Autodesk Inventor part; units mm, degrees
ref_plane "YZ Plane" through (0, 0, 0) normal (1, 0, 0) x (0, 1, 0)
ref_plane "XZ Plane" through (0, 0, 0) normal (0, 1, 0) x (-1, 0, 0)
ref_plane "XY Plane" through (0, 0, 0) normal (0, 0, 1) x (1, 0, 0)
sketch "Sketch1" plane through (0, 0, 0) normal (0, 1, 0) x (-1, 0, 0)
  line L0 (69.85, 63.5) -> (-82.55, 63.5)
  line L1 (-82.55, 63.5) -> (-82.55, -38.1)
  line L2 (-82.55, -38.1) -> (69.85, -38.1)
  line L3 (69.85, -38.1) -> (69.85, 63.5)
  circle A0 centre (25.4, -25.4) radius 3.9751
  circle A1 centre (63.5, 38.1) radius 3.175
  circle A2 centre (-76.2, 38.1) radius 3.175
  point P0 (0, 0)
  dimension "d0" = 101.6
  dimension "d1" = 152.4
  dimension "d3" = 38.1
  dimension "d4" = 7.9502
  dimension "d16" = 6.35
  dimension "d17" = 6.35
  dimension "d18" = 25.4
  dimension "d20" = 6.35
  dimension "d21" = 6.35
  dimension "d22" = 44.45
  dimension "d24" = 25.4
  dimension "d26" = 25.4
extrude "Extrusion1" add sketch "Sketch1" along normal blind 25.4
sketch "Sketch2" plane through (0, 25.4, 0) normal (0, 1, 0) x (1, 0, 0)
  circle A0 centre (6.35, -38.1) radius 16.51
  circle A1 centre (76.2, -38.1) radius 3.175
  line L0 (82.55, -63.5) -> (82.55, 38.1)
  point P0 (0, 0)
  dimension "d7" = 33.02
  dimension "d25" = 76.2
extrude "Extrusion2" add sketch "Sketch2" along normal blind 101.6 contours A0
sketch "Sketch3" plane through (6.35, 127, 38.1) normal (0, 1, 0) x (1, 0, 0)
  circle A0 centre (0, 0) radius 13.0175
  point P0 (-6.35, 38.1)
  dimension "d10" = 26.035
extrude "Extrusion3" cut sketch "Sketch3" against normal blind 41.91
sketch "Sketch4" plane through (6.35, 85.09, 38.1) normal (0, 1, 0) x (1, 0, 0)
  circle A0 centre (0, 0) radius 16.51
  circle A1 centre (0, 0) radius 16.002
  point P0 (-6.35, 38.1)
  dimension "d13" = 32.004
extrude "Extrusion4" cut sketch "Sketch4" against normal blind 59.69 contours A1
properties part number "Bottom Plate For Side to Side Motion"
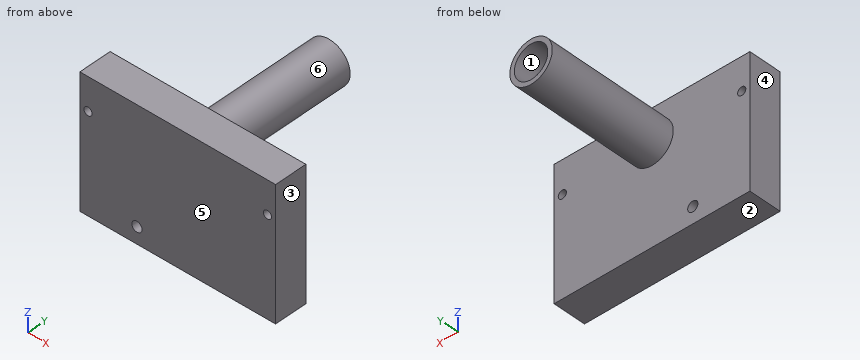
CAD build for the part. Positions are in the model's coordinates, mm. Face numbers are marked on the shaded views. A direction names the side the tool comes from. Round coordinates to 2 decimals unless told otherwise and drop trailing zeros. Order: outer loops, then holes, each group sorted by start corner. A loop starts at its lowest first (then second) coordinate and runs counter-clockwise, first axis right, second up. Notation, with made-up numbers: (18, 52) - (46, 52) arc R15 cw to (46, 70) - close; hole circle Ø10 at (-10.5, 25). An arc over 180 degrees is marked (long way). Use CSV: the item, a comma, the result in double quotes. Start each with the question number.
1) Pin check, flat tips, straight feed: pin 1 Ø9.5 at (x, z) = (4.5, 37.5) entering from +Y; pin 2 Ø2 at (x, y) = (2, 36.5) entering from -Z; pin 3 Ø5 at (y, z) = (45.5, 35.5) entering from +X. Stop position of each tip, or through.
2) Two-plate mould, pull along X, no slides. Class the marked faces 1, 2, 3 and 4: pulls with the +X half, pulls with the -X half, needs draft (parallel to the pull), parting line crosses it, or undercut.
3) Wall check: L1, parallel to X at y = 11, z = 38; L2, parallel to Z at x = -63, y = 20.5; L3, parallel to X at y = 46, z = 38. Give the ranges that are in metal, low to high. Write a range as [from, to].
4) Saw through at B-B (x = -63.5). List the corners of the cut face in (y, z) (3 decimals).
5) Saw through at A-A (z = 38.1). Count the separate pieces of the cut face and the enclosed holes in it, and give its area (3 significant figures).
6) Saw through at C-C (z = -25.4). List the corners of the cut face in (x, y).
7) Tool access for the marked faces 5 and 6: list every direction of +Z, -Z, +X, -X, +Y, -Y with a clear straight run to the whole face (end or side of a thin tool).
8) Saw through at D-D (x = 6.35). List the corners of the cut face in (y, z), and give its area (3 significant figures).
Values follow:
1,pin 1,"stops at y = 25.4"
1,pin 2,"stops at z = 21.93"
1,pin 3,"stops at x = 22.86"
2,face 1,"undercut"
2,face 2,"needs draft"
2,face 3,"pulls with the +X half"
2,face 4,"pulls with the -X half"
3,L1,"x = [-69.85, -66.67], [-60.33, 73.03], [79.37, 82.55]"
3,L2,"z = [-38.1, 34.96], [41.24, 63.5]"
3,L3,"x = [-10.16, -9.65], [22.35, 22.86]"
4,outline,"(0, -38.1) - (25.4, -38.1) - (25.4, 34.925) - (0, 34.925) - close; (0, 41.275) - (25.4, 41.275) - (25.4, 63.5) - (0, 63.5) - close"
5,separate pieces,"3"
5,enclosed holes,"0"
5,area,"3,900 mm2"
6,outline,"(-69.85, 0) - (-29.38, 0) - (-29.38, 25.4) - (-69.85, 25.4) - close; (-21.42, 0) - (82.55, 0) - (82.55, 25.4) - (-21.42, 25.4) - close"
7,face 5,"+Z, -Z, +X, -X, -Y"
7,face 6,"+Y"
8,outline,"(0, -38.1) - (25.4, -38.1) - (25.4, 21.59) - (127, 21.59) - (127, 25.08) - (85.09, 25.08) - (85.09, 22.1) - (25.4, 22.1) - (25.4, 54.1) - (85.09, 54.1) - (85.09, 51.12) - (127, 51.12) - (127, 54.61) - (25.4, 54.61) - (25.4, 63.5) - (0, 63.5) - close"
8,area,"2,930 mm2"
